Source: CAD feature listing. Evaluate the final solid. Frame: model axes, mm. Face numbers are marked on the shaded views. A direction names the side the tool comes from. Give positions to 0.01 mm unless a question says otherwise; leave off trailing zeros. Order: outer loops, then holes, each group sorted by start corner. A loop starts at its lowest first (then second) coordinate and runs counter-clockwise, first axis right, second up.
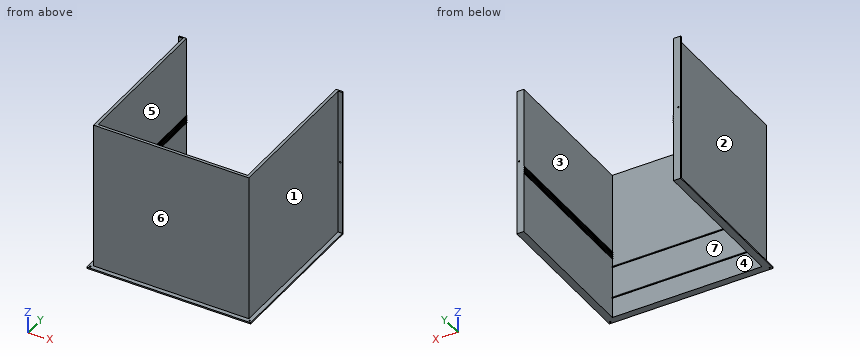
from build123d import *

# Parameters (mm, degrees)
BOSS_EXTRUDE1_DEPTH = 526.6975777
SKETCH2_W           = 526.6975777
SKETCH2_H           = 3
BOSS_EXTRUDE2_DEPTH = 2
SKETCH3_W           = 2.2
SKETCH3_H           = 2
BOSS_EXTRUDE3_DEPTH = 526.6975777
SKETCH4_R           = 2.5
BOSS_EXTRUDE4_DEPTH = 5
SKETCH5_W           = 15
SKETCH5_H           = 521.6975777
SKETCH5_R           = 2.5
BOSS_EXTRUDE5_DEPTH = 5


with BuildPart() as part:
    # Sketch1 → Boss-Extrude1 (new body)
    with BuildSketch(Plane.XY):
        Polygon((-263.34878885, -263.34878885), (263.34878885, -263.34878885), (263.34878885, 263.34878885), (273.34878885, 263.34878885), (273.34878885, -273.34878885), (-273.34878885, -273.34878885), (-273.34878885, 263.34878885), (-263.34878885, 263.34878885), align=None)
    extrude(amount=BOSS_EXTRUDE1_DEPTH)

    # Sketch2 → Boss-Extrude2 (add)
    with BuildSketch(Plane(origin=(0, -263.34878885, 0), x_dir=(1, 0, 0), z_dir=(0, 1, 0))):
        with Locations((0, -72.401892101)):
            Rectangle(SKETCH2_W, SKETCH2_H)
        with Locations((0, -186.401892101)):
            Rectangle(SKETCH2_W, SKETCH2_H)
    extrude(amount=BOSS_EXTRUDE2_DEPTH)

    # Sketch3 → Boss-Extrude3 (add)
    with BuildSketch(Plane(origin=(0, -263.34878885, 0), x_dir=(1, 0, 0), z_dir=(0, 1, 0))):
        with Locations((-262.24878885, -217.20163133)):
            Rectangle(SKETCH3_W, SKETCH3_H)
        with Locations((-262.24878885, -224.70163133)):
            Rectangle(SKETCH3_W, SKETCH3_H)
        with Locations((262.24878885, -224.70163133)):
            Rectangle(SKETCH3_W, SKETCH3_H)
        with Locations((262.24878885, -217.20163133)):
            Rectangle(SKETCH3_W, SKETCH3_H)
    boss_extrude3 = extrude(amount=BOSS_EXTRUDE3_DEPTH)

    # Mirror1: Boss-Extrude3 across plane
    add(boss_extrude3.mirror(Plane.XY.offset(228.70163133)))

    # Sketch4 → Boss-Extrude4 (add)
    with BuildSketch(Plane(origin=(0, 0, 0), x_dir=(-1, 0, 0), z_dir=(0, 0, -1))):
        Polygon((-263.34878885, 263.34878885), (-263.34878885, -263.34878885), (263.34878885, -263.34878885), (263.34878885, 263.34878885), (288.34878885, 263.34878885), (288.34878885, -288.34878885), (-288.34878885, -288.34878885), (-288.34878885, 263.34878885), align=None)
        with Locations((-280.84878885, -280.84878885)):
            Circle(SKETCH4_R, mode=Mode.SUBTRACT)
        with Locations((280.84878885, -280.84878885)):
            Circle(SKETCH4_R, mode=Mode.SUBTRACT)
    extrude(amount=-BOSS_EXTRUDE4_DEPTH)

    # Sketch5 → Boss-Extrude5 (add)
    # profile 1 of 2: a face of its own
    with BuildSketch(Plane(origin=(0, 263.34878885, 0), x_dir=(1, 0, 0), z_dir=(0, 1, 0))):
        with Locations((-280.84878885, -265.84878885)):
            Rectangle(SKETCH5_W, SKETCH5_H)
        with Locations(Location((-280.704595135, -265.84878885, 0), (0, 0, 270))):
            Circle(SKETCH5_R, mode=Mode.SUBTRACT)
    # profile 2 of 2: a face of its own
    with BuildSketch(Plane(origin=(0, 263.34878885, 0), x_dir=(1, 0, 0), z_dir=(0, 1, 0))):
        with Locations((280.84878885, -265.84878885)):
            Rectangle(SKETCH5_W, SKETCH5_H)
        with Locations(Location((280.704595135, -265.84878885, 0), (0, 0, 90))):
            Circle(SKETCH5_R, mode=Mode.SUBTRACT)
    extrude(amount=-BOSS_EXTRUDE5_DEPTH)


solid = part.part
1) First-contact query: pin 1 Ø10 at (x, z) = (143, 185) entering from +Y; pin 2 Ø2 at (x, y) = (-122, -262) entering from +Z; pin 3 Ø1.8 at (x, y) = (262, -108) entering from -Z; pin 4 Ø3 at (x, y) = (-280.85, -280.85) entering from -Z. Flat tips, straight axial feed; report the tip coordinate or a pass-through.
Checks:
pin 1: stops at y = -261.35
pin 2: stops at z = 187.9
pin 3: stops at z = 216.2
pin 4: passes through
2) Section query A-A on z = 443.5. Output: boundary loops of the cut face in (x, y), and give its area (3 significant figures).
Checks:
outline: (-288.35, 258.35) - (-273.35, 258.35) - (-273.35, -273.35) - (273.35, -273.35) - (273.35, 258.35) - (288.35, 258.35) - (288.35, 263.35) - (263.35, 263.35) - (263.35, -263.35) - (-263.35, -263.35) - (-263.35, 263.35) - (-288.35, 263.35) - close
area: 16,200 mm2
3) Ray query, L1, parallel to X at y = 147.5, z = 294; L2, parallel to Y at x = -178, z = 66; L3, parallel to X at y = -133, z = 232. Return the intervals inside material, ascending.
Checks:
L1: x = -273.35 to -263.35, 263.35 to 273.35
L2: y = -273.35 to -263.35
L3: x = -273.35 to -261.15, 261.15 to 273.35
4) Section query B-B on x = 140. Output: boundary loops of the cut face in (y, z).
Checks:
outline: (-288.35, 0) - (-263.35, 0) - (-263.35, 70.9) - (-261.35, 70.9) - (-261.35, 73.9) - (-263.35, 73.9) - (-263.35, 184.9) - (-261.35, 184.9) - (-261.35, 187.9) - (-263.35, 187.9) - (-263.35, 526.7) - (-273.35, 526.7) - (-273.35, 5) - (-288.35, 5) - close
5) Reachability of the marked faces 4, 5, 6 and 7 from +Z, -Z, +X, -X, +Y, -Y: full face, straight path, thin tool, end or side. Return the list, or none.
Checks:
face 4: -Z, +Y
face 5: +Z, +Y
face 6: +Z, +X, -X, -Y
face 7: +Y
6) Pull-direction query (X, two-part tool) for the marked faces 1, 2 and 3; classes: +X half, -X half, draft (parallel to the pull), parting line (faces both ways), or undercut.
Checks:
face 1: +X half
face 2: -X half
face 3: undercut
